Build history of the part. All positions in model axes, mm. A direction names the side the tool comes from. Coordinates: 2 decimals unless noted, no trailing zeros. Order: outer loops, then holes, each group sorted by start corner. A loop starts at its lowest first (then second) coordinate and runs counter-clockwise, first axis right, second up. Notation, with made-up numbers: M 16.25,54.25 L 20.25,54.25 A9 ccw 20.25,64.25 Z; hole C 47.25,3.5 d1. An arc over 180 degrees is marked long. Write item = value, one per line. Start each with the question number.
Q1. Pin check, flat tips, straight feed: P1, Ø5, axis at y = 7, z = 8.5, coming from the +X side; P2, Ø1, axis at x = -11.5, y = 3.5, coming from the -Z side; P3, Ø6, axis at y = 2.5, z = -12.5, coming from the -X side. Stop position of each tip, or through.
Q2. Band-saw the part on A-A on z = 0. Write the cut outline in (x, y) (3 decimals), plus the area to 3 significant figures.
Q3. Band-saw the part on B-B on x = 0. Write the cut outline in (y, z) (3 decimals).
Q4. Band-saw the part on C-C on y = 4.25. Write the cut outline in (x, z) (3 decimals).
Q5. Drill centre lines: probe 1 along X at (y, z) = (5.75, 0.5); probe 2 along X at (y, z) = (11.5, 1.5). Where is each one in solid material? Low to high.
Q6. 3-axis set-ups, long thin cutter, end or side, ignore diameter. For faces 1 (the face through (3, 6, 0)), 2 (the face through (3.3, 13, 0.2)), 3 (the face through (-1.85, 2.535, 7.644)): which of +Z, -Z, +X, -X, +Y, -Y reach the whole face in a straight line?
Q7. Band-saw the part on D-D on x = 10.5. Write the cut outline in (y, z).
Q8. Pull direction X, two halves, no side cores. Call faces 4 (the face through (-3.441, 6.409, -15.497)), 5 (the face through (3.3, 0, 0.2)), 6 (the face through (7.647, 2.535, -1.893)): released by +X, released by -X, zero draft, split by the parting line, or undercut.
```python
from build123d import *

# Parameters (mm, degrees)
F0_R           = 15.875
F1_DEPTH       = 13
F2_W           = 6
F2_H           = 6
F3_DEPTH       = 13.001
F6_D           = 1
F6_DEPTH       = 5
F6_TIP         = 0.3004303095
F6_ON_F5_D     = 1
F6_ON_F5_DEPTH = 5
F6_ON_F5_TIP   = 0.3004303095


with BuildPart() as f1:
    # F0 (on Front) → F1 (new body)
    with BuildSketch(Plane.XZ):
        Circle(F0_R)
    extrude(amount=-F1_DEPTH)

    # F2 (on Front) → F3 (cut, through all)
    with BuildSketch(Plane.XZ):
        Rectangle(F2_W, F2_H)
    extrude(amount=-F3_DEPTH, mode=Mode.SUBTRACT)

    # F6
    with Locations(Plane.XZ):
        with Locations((9.4752308679, 9.4752308679), (3.4681752044, -12.9434060723), (-12.9434060723, 3.4681752044)):
            Hole(F6_D / 2, depth=F6_DEPTH)
            with Locations((0, 0, -(F6_DEPTH + F6_TIP / 2))):  # 118° drill point
                Cone(0, F6_D / 2, F6_TIP, mode=Mode.SUBTRACT)

    # F6 on F5
    with Locations(Plane.XZ):
        with Locations((-1.9152609338, 7.1478511145), (7.1478511145, -1.9152609338), (-5.2325901808, -5.2325901808)):
            Hole(F6_ON_F5_D / 2, depth=F6_ON_F5_DEPTH)
            with Locations((0, 0, -(F6_ON_F5_DEPTH + F6_ON_F5_TIP / 2))):  # 118° drill point
                Cone(0, F6_ON_F5_D / 2, F6_ON_F5_TIP, mode=Mode.SUBTRACT)


solid = f1.part
```
Recorded:
q1.P1 = 14.7
q1.P2 = -11.45
q1.P3 = -12.72
q2.outline = M -15.875,0 L -3,0 L -3,13 L -15.875,13 Z; M 3,0 L 15.875,0 L 15.875,13 L 3,13 Z
q2.area = 335 mm2
q3.outline = M 0,-15.875 L 13,-15.875 L 13,-3 L 0,-3 Z; M 0,3 L 13,3 L 13,15.875 L 0,15.875 Z
q4.outline = C 0,0 d31.75; hole C -12.943,3.468 d1; hole C -5.233,-5.233 d1; hole M -3,-3 L 3,-3 L 3,3 L -3,3 Z; hole C -1.915,7.148 d1; hole C 3.468,-12.943 d1; hole C 7.148,-1.915 d1; hole C 9.475,9.475 d1
q5.probe_1 = -15.87 to -3, 3 to 15.87
q5.probe_2 = -15.8 to -3, 3 to 15.8
q6.face_1 = +Y, -Y
q6.face_2 = +Z, -Z, +X, -X, +Y
q6.face_3 = -Y
q7.outline = M 0,-11.91 L 13,-11.91 L 13,11.91 L 0,11.91 Z
q8.face_4 = split by the parting line
q8.face_5 = zero draft
q8.face_6 = undercut
